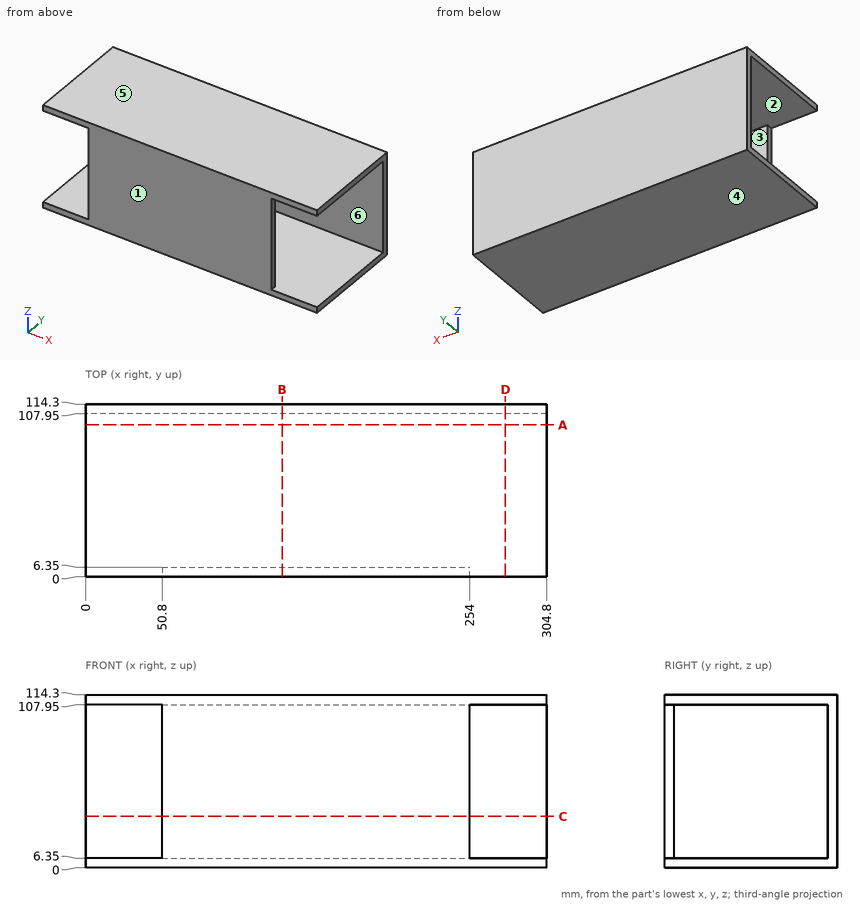
Job drawing, mm, ordinate dimensions from the low corner. One solid piece. A direction names the side the tool comes from. Give positions to 0.01 mm unless a question says otherwise; leave off trailing zeros. Write each loop counter-clockwise with the first axis right and the second up, starting at its lowest first coordinate (ties: lowest second). Pieces come first, ordered by that corner, then holes. Notation, with made-up numbers: M -16,67 L 2,67 A20 cw 2,95 Z; hole C -31.75,-8 d6. An arc over 180 degrees is marked long. One line per item, written item: value. Start each with the question number.
Q1. 3-axis set-ups, long thin cutter, end or side, ignore diameter. For the marked faces 5 and 6: which of +Z, -Z, +X, -X, +Y, -Y reach the whole face in a straight line?
Q2. Saw through at C-C, the plane z = 34. Write the cut outline in (x, y).
Q3. Saw through at D-D, the plane x = 277.5. Write the cut outline in (y, z).
Q4. Drop flat-ended pins along their axis: pin 1 Ø1.9 at (y, z) = (2.5, 60.5) entering from +X; pin 2 Ø3 at (y, z) = (2, 48.5) entering from -X. Give the stop position or say it passes through.
Q5. Saw through at B-B, the plane x = 130. Write the cut outline in (y, z).
Q6. Saw through at A-A, the plane y = 100.5. Write the cut outline in (x, z), plus the area to 3 significant figures.
Q7. Two-plate mould, pull along Z, no slides. Class the marked faces 1, 2, 3 and 4: +Z half, -Z half, draft (parallel to the pull), parting line (faces both ways), or undercut.
Q8. Probe probe 1 along Z at (x, y) = (142.5, 19); probe 2 along Y at (x, z) = (284, 49.5). List the from-to ranges inside material, lowest first. Write a range as [from, to].
Output values:
1. face 5: +Z, +X, -X, +Y, -Y
1. face 6: +X, -X
2. outline: M 0,107.95 L 304.8,107.95 L 304.8,114.3 L 0,114.3 Z; M 50.8,0 L 254,0 L 254,6.35 L 50.8,6.35 Z
3. outline: M 0,0 L 114.3,0 L 114.3,114.3 L 0,114.3 L 0,107.95 L 107.95,107.95 L 107.95,6.35 L 0,6.35 Z
4. pin 1: stops at x = 254
4. pin 2: stops at x = 50.8
5. outline: M 0,0 L 114.3,0 L 114.3,114.3 L 0,114.3 Z; hole M 6.35,6.35 L 107.95,6.35 L 107.95,107.95 L 6.35,107.95 Z
6. outline: M 0,0 L 304.8,0 L 304.8,6.35 L 0,6.35 Z; M 0,107.95 L 304.8,107.95 L 304.8,114.3 L 0,114.3 Z
6. area: 3,870 mm²
7. face 1: draft
7. face 2: undercut
7. face 3: undercut
7. face 4: -Z half
8. probe 1: z = [0, 6.35], [107.95, 114.3]
8. probe 2: y = [107.95, 114.3]
